from build123d import *

# Parameters (mm, degrees)
SKETCH1_R           = 50.8
SKETCH1_R_2         = 12.7
SKETCH1_R_3         = 2.921
BOSS_EXTRUDE2_DEPTH = 25.4
SKETCH2_R           = 44.45
CUT_EXTRUDE1_DEPTH  = 19.05


with BuildPart() as part:
    # Sketch1 → Boss-Extrude2 (new body)
    with BuildSketch(Plane.XY):
        Circle(SKETCH1_R)
        Circle(SKETCH1_R_2, mode=Mode.SUBTRACT)
        with Locations((0, 20.32)):
            Circle(SKETCH1_R_3, mode=Mode.SUBTRACT)
        with Locations((19.325468411, 6.279225326)):
            Circle(SKETCH1_R_3, mode=Mode.SUBTRACT)
        with Locations((11.943796327, -16.439225326)):
            Circle(SKETCH1_R_3, mode=Mode.SUBTRACT)
        with Locations((-11.943796327, -16.439225326)):
            Circle(SKETCH1_R_3, mode=Mode.SUBTRACT)
        with Locations((-19.325468411, 6.279225326)):
            Circle(SKETCH1_R_3, mode=Mode.SUBTRACT)
    extrude(amount=BOSS_EXTRUDE2_DEPTH)

    # Sketch2 → Cut-Extrude1 (cut)
    with BuildSketch(Plane.XY.offset(25.4)):
        Circle(SKETCH2_R)
    extrude(amount=-CUT_EXTRUDE1_DEPTH, mode=Mode.SUBTRACT)


solid = part.part
The listing builds one solid part. Answer for the finished solid, in the listing's coordinates (mm). A direction names the side the tool comes from. Give positions to 0.01 mm unless a question says otherwise; leave off trailing zeros. Write each loop counter-clockwise with the first axis right and the second up, starting at its lowest first coordinate (ties: lowest second). Pieces come first, ordered by that corner, then holes. Notation, with made-up numbers: (54, 24) -> (65, 24) arc R31 cw to (65, 63) -> close; hole circle Ø2 at (22.5, 50). An arc over 180 degrees is marked (long way). Use a Markdown table: item, result.
(1) Section A-A, the plane x = 0 is taken. Determine the outline of the cut face in (y, z), then the cut area to 3 significant figures.
Return value:
| item | result |
|---|---|
| outline | (-50.8, 0) -> (-12.7, 0) -> (-12.7, 6.35) -> (-44.45, 6.35) -> (-44.45, 25.4) -> (-50.8, 25.4) -> close; (12.7, 0) -> (17.4, 0) -> (17.4, 6.35) -> (12.7, 6.35) -> close; (23.24, 0) -> (50.8, 0) -> (50.8, 25.4) -> (44.45, 25.4) -> (44.45, 6.35) -> (23.24, 6.35) -> close |
| area | 689 mm2 |
(2) Flat-ended cylindrical pins translate along their axes: P1, Ø4.5, axis at x = 19.33, y = 6.28, coming from the -Z side; P2, Ø10, axis at x = -16.5, z = 15.5, coming from the +Y side; P3, Ø8, axis at x = -17.5, z = 22, coming from the -Y side; P4, Ø12, axis at x = 32, z = 8.5, coming from the +Y side. Find the tip coordinate at first contact, or state that the pin passes through.
Return value:
| item | result |
|---|---|
| P1 | through |
| P2 | y = 49.48 |
| P3 | y = -48.97 |
| P4 | y = 43.64 |
(3) Section B-B, the plane y = 0 is taken. Determine the outline of the cut face in (x, z).
Return value:
| item | result |
|---|---|
| outline | (-50.8, 0) -> (-12.7, 0) -> (-12.7, 6.35) -> (-44.45, 6.35) -> (-44.45, 25.4) -> (-50.8, 25.4) -> close; (12.7, 0) -> (50.8, 0) -> (50.8, 25.4) -> (44.45, 25.4) -> (44.45, 6.35) -> (12.7, 6.35) -> close |
(4) Find the intervals of material crossed by probe 1 along Y at (x, z) = (0, 4.25); probe 2 along Y at (x, z) = (0, 10.5); probe 3 along X at (y, z) = (37.5, 24), in increasing order. Write a range as from..to.
Return value:
| item | result |
|---|---|
| probe 1 | -50.8..-12.7, 12.7..17.4, 23.24..50.8 |
| probe 2 | -50.8..-44.45, 44.45..50.8 |
| probe 3 | -34.27..-23.87, 23.87..34.27 |
(5) Section D-D, the plane z = 3.5 is taken. Determine the outline of the cut face in (x, y).
Return value:
| item | result |
|---|---|
| outline | circle Ø101.6 at (0, 0); hole circle Ø5.84 at (-19.33, 6.28); hole circle Ø5.84 at (-11.94, -16.44); hole circle Ø25.4 at (0, 0); hole circle Ø5.84 at (0, 20.32); hole circle Ø5.84 at (11.94, -16.44); hole circle Ø5.84 at (19.33, 6.28) |
(6) Section C-C, the plane x = 20.5 is taken. Determine the outline of the cut face in (y, z), then the cut area to 3 significant figures.
Return value:
| item | result |
|---|---|
| outline | (-46.48, 0) -> (3.6, 0) -> (3.6, 6.35) -> (-39.44, 6.35) -> (-39.44, 25.4) -> (-46.48, 25.4) -> close; (8.95, 0) -> (46.48, 0) -> (46.48, 25.4) -> (39.44, 25.4) -> (39.44, 6.35) -> (8.95, 6.35) -> close |
| area | 825 mm2 |
(7) For faces 1 (the cylindrical face through (-12.58, -19.29, 3.13)), 2 (the flat face through (9.3, -9.3, 6.35)), determine the directions among +Z, -Z, +X, -X, +Y, -Y from which every point of the face is accessible in a straight line to the end or side of a thin tool.
Return value:
| item | result |
|---|---|
| face 1 | +Z, -Z |
| face 2 | +Z |
(8) Determine the mould class of faces 3 (the cylindrical face through (42.397, 13.352, 16.008)), 4 (the flat face through (0, -45, 25.4)), 5 (the cylindrical face through (-11.012, -49.592, 12.522)) for opening direction X: released by +X, released by -X, zero draft, split by the parting line, or undercut.
Return value:
| item | result |
|---|---|
| face 3 | undercut |
| face 4 | zero draft |
| face 5 | split by the parting line |
